Design review of the part built by this model. Coordinates are the model's own, in mm. Give positions to 0.01 mm unless a question says otherwise; leave off trailing zeros.
```python
from build123d import *

# Parameters (mm, degrees)
F0_W     = 95
F0_H     = 95
F0_R     = 1.5
F1_DEPTH = 1


with BuildPart() as f1:
    # F0 (on Top) → F1 (new body)
    with BuildSketch(Plane.XY):
        Rectangle(F0_W, F0_H)
        with Locations((-44.5, -44.75)):
            Circle(F0_R, mode=Mode.SUBTRACT)
        with Locations((-31.75, -44.75)):
            Circle(F0_R, mode=Mode.SUBTRACT)
        with Locations((-44.5, -32)):
            Circle(F0_R, mode=Mode.SUBTRACT)
        with Locations((-31.75, -32)):
            Circle(F0_R, mode=Mode.SUBTRACT)
        with Locations((-19, -44.75)):
            Circle(F0_R, mode=Mode.SUBTRACT)
        with Locations((-6.25, -44.75)):
            Circle(F0_R, mode=Mode.SUBTRACT)
        with Locations((-19, -32)):
            Circle(F0_R, mode=Mode.SUBTRACT)
        with Locations((-6.25, -32)):
            Circle(F0_R, mode=Mode.SUBTRACT)
        with Locations((-44.5, -19.25)):
            Circle(F0_R, mode=Mode.SUBTRACT)
        with Locations((-31.75, -19.25)):
            Circle(F0_R, mode=Mode.SUBTRACT)
        with Locations((-44.5, -6.5)):
            Circle(F0_R, mode=Mode.SUBTRACT)
        with Locations((-31.75, -6.5)):
            Circle(F0_R, mode=Mode.SUBTRACT)
        with Locations((-19, -19.25)):
            Circle(F0_R, mode=Mode.SUBTRACT)
        with Locations((-6.25, -19.25)):
            Circle(F0_R, mode=Mode.SUBTRACT)
        with Locations((-19, -6.5)):
            Circle(F0_R, mode=Mode.SUBTRACT)
        with Locations((-6.25, -6.5)):
            Circle(F0_R, mode=Mode.SUBTRACT)
        with Locations((6.5, -44.75)):
            Circle(F0_R, mode=Mode.SUBTRACT)
        with Locations((19.25, -44.75)):
            Circle(F0_R, mode=Mode.SUBTRACT)
        with Locations((6.5, -32)):
            Circle(F0_R, mode=Mode.SUBTRACT)
        with Locations((19.25, -32)):
            Circle(F0_R, mode=Mode.SUBTRACT)
        with Locations((32, -44.75)):
            Circle(F0_R, mode=Mode.SUBTRACT)
        with Locations((44.75, -44.75)):
            Circle(F0_R, mode=Mode.SUBTRACT)
        with Locations((32, -32)):
            Circle(F0_R, mode=Mode.SUBTRACT)
        with Locations((44.75, -32)):
            Circle(F0_R, mode=Mode.SUBTRACT)
        with Locations((6.5, -19.25)):
            Circle(F0_R, mode=Mode.SUBTRACT)
        with Locations((19.25, -19.25)):
            Circle(F0_R, mode=Mode.SUBTRACT)
        with Locations((6.5, -6.5)):
            Circle(F0_R, mode=Mode.SUBTRACT)
        with Locations((19.25, -6.5)):
            Circle(F0_R, mode=Mode.SUBTRACT)
        with Locations((32, -19.25)):
            Circle(F0_R, mode=Mode.SUBTRACT)
        with Locations((44.75, -19.25)):
            Circle(F0_R, mode=Mode.SUBTRACT)
        with Locations((32, -6.5)):
            Circle(F0_R, mode=Mode.SUBTRACT)
        with Locations((44.75, -6.5)):
            Circle(F0_R, mode=Mode.SUBTRACT)
        with Locations((-44.5, 6.25)):
            Circle(F0_R, mode=Mode.SUBTRACT)
        with Locations((-31.75, 6.25)):
            Circle(F0_R, mode=Mode.SUBTRACT)
        with Locations((-44.5, 19)):
            Circle(F0_R, mode=Mode.SUBTRACT)
        with Locations((-31.75, 19)):
            Circle(F0_R, mode=Mode.SUBTRACT)
        with Locations((-19, 6.25)):
            Circle(F0_R, mode=Mode.SUBTRACT)
        with Locations((-6.25, 6.25)):
            Circle(F0_R, mode=Mode.SUBTRACT)
        with Locations((-19, 19)):
            Circle(F0_R, mode=Mode.SUBTRACT)
        with Locations((-6.25, 19)):
            Circle(F0_R, mode=Mode.SUBTRACT)
        with Locations((-44.5, 31.75)):
            Circle(F0_R, mode=Mode.SUBTRACT)
        with Locations((-31.75, 31.75)):
            Circle(F0_R, mode=Mode.SUBTRACT)
        with Locations((-44.5, 44.5)):
            Circle(F0_R, mode=Mode.SUBTRACT)
        with Locations((-31.75, 44.5)):
            Circle(F0_R, mode=Mode.SUBTRACT)
        with Locations((-19, 31.75)):
            Circle(F0_R, mode=Mode.SUBTRACT)
        with Locations((-6.25, 31.75)):
            Circle(F0_R, mode=Mode.SUBTRACT)
        with Locations((-19, 44.5)):
            Circle(F0_R, mode=Mode.SUBTRACT)
        with Locations((-6.25, 44.5)):
            Circle(F0_R, mode=Mode.SUBTRACT)
        with Locations((6.5, 6.25)):
            Circle(F0_R, mode=Mode.SUBTRACT)
        with Locations((19.25, 6.25)):
            Circle(F0_R, mode=Mode.SUBTRACT)
        with Locations((6.5, 19)):
            Circle(F0_R, mode=Mode.SUBTRACT)
        with Locations((19.25, 19)):
            Circle(F0_R, mode=Mode.SUBTRACT)
        with Locations((32, 6.25)):
            Circle(F0_R, mode=Mode.SUBTRACT)
        with Locations((44.75, 6.25)):
            Circle(F0_R, mode=Mode.SUBTRACT)
        with Locations((32, 19)):
            Circle(F0_R, mode=Mode.SUBTRACT)
        with Locations((44.75, 19)):
            Circle(F0_R, mode=Mode.SUBTRACT)
        with Locations((6.5, 31.75)):
            Circle(F0_R, mode=Mode.SUBTRACT)
        with Locations((19.25, 31.75)):
            Circle(F0_R, mode=Mode.SUBTRACT)
        with Locations((6.5, 44.5)):
            Circle(F0_R, mode=Mode.SUBTRACT)
        with Locations((19.25, 44.5)):
            Circle(F0_R, mode=Mode.SUBTRACT)
        with Locations((32, 31.75)):
            Circle(F0_R, mode=Mode.SUBTRACT)
        with Locations((44.75, 31.75)):
            Circle(F0_R, mode=Mode.SUBTRACT)
        with Locations((32, 44.5)):
            Circle(F0_R, mode=Mode.SUBTRACT)
        with Locations((44.75, 44.5)):
            Circle(F0_R, mode=Mode.SUBTRACT)
    extrude(amount=F1_DEPTH)


solid = f1.part
```
1. For pin 1 (3.5 mm diameter, centred on x = -44.5, y = 44.5, fed in from +Z); pin 2 (2.5 mm diameter, centred on x = 44.75, y = 44.5, fed in from -Z), all flat-tipped, find the tip position at first contact; note any pin that passes through.
Recorded:
pin 1: stops at z = 1
pin 2: passes through
2. Draft analysis for pull direction Y (two halves, no side actions). For faces 1 (the face through (-6.575, 43.036, 0.493)), 2 (the face through (-1, 1, 1)), state which applies: pulls with the +Y half, pulls with the -Y half, needs draft (parallel to the pull), parting line crosses it, or undercut.
Recorded:
face 1: undercut
face 2: needs draft
3. Take a section at A-A (x = 32). State how many separate pieces and enclosed holes the cut face has, then the cut area to 3 significant figures.
Recorded:
separate pieces: 9
enclosed holes: 0
area: 71.0 mm2
